The listing builds one solid part. Answer for the finished solid, in the listing's coordinates (mm). A direction names the side the tool comes from. Give positions to 0.01 mm unless a question says otherwise; leave off trailing zeros. Order: outer loops, then holes, each group sorted by start corner. A loop starts at its lowest first (then second) coordinate and runs counter-clockwise, first axis right, second up. Notation, with made-up numbers: (36, -11.5) - (90, -11.5) arc R28 cw to (90, 8.5) - close; hole circle Ø11 at (-29.75, 80.25). An arc over 180 degrees is marked (long way). Answer in a Markdown table with one row per item. Add a question column.
```python
from build123d import *

# Parameters (mm, degrees)
SKETCH_1_R          = 10.5
SKETCH_1_R_2        = 7.5
EXTRUDE_1_DEPTH     = 12
SKETCH_2_R          = 13.5
SKETCH_2_R_2        = 10.5
EXTRUDE_2_DEPTH     = 3.9
SKETCH_3_W          = 25.92950511
SKETCH_3_H          = 4
CUT_EXTRUDE_1_DEPTH = 4


with BuildPart() as part:
    # 草图1 → 拉伸-薄壁1 (new body)
    with BuildSketch(Plane.XY):
        Circle(SKETCH_1_R)
        Circle(SKETCH_1_R_2, mode=Mode.SUBTRACT)
    extrude(amount=EXTRUDE_1_DEPTH)

    # 草图2 → 拉伸-薄壁2 (add)
    with BuildSketch(Plane(origin=(0, 0, 0), x_dir=(-1, 0, 0), z_dir=(0, 0, -1))):
        Circle(SKETCH_2_R)
        Circle(SKETCH_2_R_2, mode=Mode.SUBTRACT)
    extrude(amount=-EXTRUDE_2_DEPTH)

    # 草图3 → 切除-拉伸1 (cut)
    with BuildSketch(Plane.XY.offset(12)):
        Rectangle(SKETCH_3_W, SKETCH_3_H)
    extrude(amount=-CUT_EXTRUDE_1_DEPTH, mode=Mode.SUBTRACT)


solid = part.part
```
(1) Find section B-B, the plane x = 0. Write down the section's boundary in (y, z).
(2) Find section C-C, the plane z = 8.5. Write down the section's boundary in (x, y), plus the area to 3 significant figures.
(3) Straight lines are drawn through the part: line 1 (Y direction, x = 0, z = 6); line 2 (Y direction, x = 0, z = 2.5). For each, find the intervals that lie inside material, in ascending order.
(4) For faces 1 (the face through (6.93, -2.87, 5.92)), 2 (the face through (10, 3.2, 7.9)), 3 (the face through (9, 0, 8)), determine the directions among +Z, -Z, +X, -X, +Y, -Y from which every point of the face is accessible in a straight line to the end or side of a thin tool.
(5) Find section A-A, the plane y = 0. Write down the section's boundary in (x, z).
(6) Find section D-D, the plane y = -9.5. Write down the section's boundary in (x, z).
(7) Each of these flat-tipped pins is pushed along its axis until it touches: P1, Ø1.5, axis at x = -10, z = 7, coming from the +Y side; P2, Ø2.5, axis at x = -9.5, z = 9, coming from the +Y side; P3, Ø1.5, axis at y = 7, z = 7, coming from the -X side; P4, Ø13.5, axis at x = 0, y = 0, coming from the +Z side. Where does it stop, or does it pass through?
Answer key:
| question | item | result |
|---|---|---|
| 1 | outline | (-13.5, 0) - (-7.5, 0) - (-7.5, 12) - (-10.5, 12) - (-10.5, 3.9) - (-13.5, 3.9) - close; (7.5, 0) - (13.5, 0) - (13.5, 3.9) - (10.5, 3.9) - (10.5, 12) - (7.5, 12) - close |
| 2 | outline | (-10.31, -2) arc R10.5 ccw to (10.31, -2) - (7.23, -2) arc R7.5 cw to (-7.23, -2) - close; (-10.31, 2) - (-7.23, 2) arc R7.5 cw to (7.23, 2) - (10.31, 2) arc R10.5 ccw to start |
| 2 | area | 145 mm² |
| 3 | line 1 | -10.5 to -7.5, 7.5 to 10.5 |
| 3 | line 2 | -13.5 to -7.5, 7.5 to 13.5 |
| 4 | face 1 | +Z, -Z |
| 4 | face 2 | +Z |
| 4 | face 3 | +Z, +X, -X |
| 5 | outline | (-13.5, 0) - (-7.5, 0) - (-7.5, 8) - (-10.5, 8) - (-10.5, 3.9) - (-13.5, 3.9) - close; (7.5, 0) - (13.5, 0) - (13.5, 3.9) - (10.5, 3.9) - (10.5, 8) - (7.5, 8) - close |
| 6 | outline | (-9.59, 0) - (9.59, 0) - (9.59, 3.9) - (4.47, 3.9) - (4.47, 12) - (-4.47, 12) - (-4.47, 3.9) - (-9.59, 3.9) - close |
| 7 | P1 | y = 4.97 |
| 7 | P2 | y = 6.5 |
| 7 | P3 | x = -8.44 |
| 7 | P4 | through |
